from build123d import *

# Parameters (mm, degrees)
SKETCH2_R   = 9.525
SKETCH2_R_2 = 7.874


with BuildPart() as part:
    # Sweep1: sweep along a path in Sketch1
    with BuildLine(Plane.XY) as sweep1_path:
        Line((-82.715438584, 8.125207387), (-58.051554514, 8.125207387))
        ThreePointArc((-58.051554514, 8.125207387), (-44.819563376, 6.967558166), (-31.989619593, 3.529785091))
        Line((-31.989619593, 3.529785091), (83.882345193, -38.644161077))
        ThreePointArc((83.882345193, -38.644161077), (96.712288976, -42.081934153), (109.944280114, -43.239583374))
        Line((109.944280114, -43.239583374), (304.690435721, -43.239583374))
        ThreePointArc((304.690435721, -43.239583374), (324.412446958, -40.643131337), (342.790435721, -33.030719142))
        Line((342.790435721, -33.030719142), (363.602993383, -21.014583374))
    # Sketch2 → Sweep1 (sweep)
    with BuildSketch(Plane(origin=(-82.715438584, 8.125207387, 0), x_dir=(0, 0, -1), z_dir=(1, 0, 0))):
        Circle(SKETCH2_R)
        Circle(SKETCH2_R_2, mode=Mode.SUBTRACT)
    sweep(path=sweep1_path.line)


solid = part.part
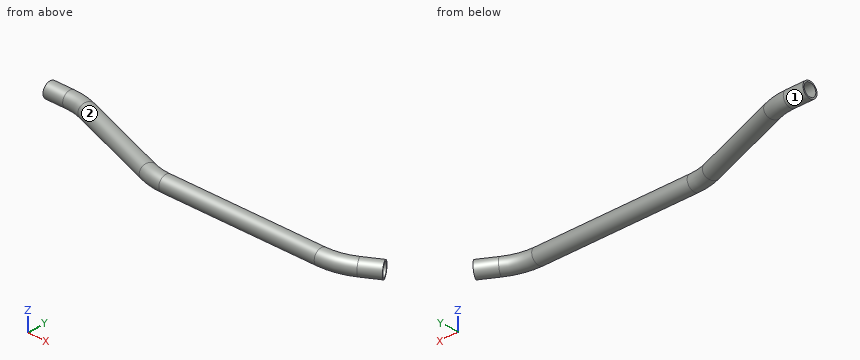
Read the model definition and answer for the solid it produces. Units are mm, in the model's axes. Face numbers are marked on the shaded views. Give positions to 0.01 mm unless a question says otherwise; leave off trailing zeros. Loops run counter-clockwise (first coordinate to the right, second up) from the corner with the lowest first, then second, coordinate; pieces in that order, holes last. Notation, with made-up numbers: (-31, -28.75) -> (-26, -28.75) arc R33 cw to (-26, 4.25) -> close; hole circle Ø7 at (0.5, 69). An arc over 180 degrees is marked (long way). Use a Markdown table: item, result.
Q1. Each of these flat-tipped pins is pushed along its axis until it touches: pin 1 (1.5 mm diameter, centred on x = 320.5, z = 0, fed in from -Y); pin 2 (2 mm diameter, centred on y = -41, z = -4, fed in from +X); pin 3 (1 mm diameter, centred on x = -22.5, z = 4.5, fed in from -Y). Where does it stop, or does it pass through?
Solved:
| item | result |
|---|---|
| pin 1 | stops at y = -51.43 |
| pin 2 | stops at x = 348.21 |
| pin 3 | stops at y = -9.18 |
Q2. Find the intervals of material crossed by line 1 along Y through (x, z) = (-72.25, 0); line 2 along Z through (x, y) = (111.5, -43); line 3 along Y through (x, z) = (262.5, 0), in increasing order.
Solved:
| item | result |
|---|---|
| line 1 | y = -1.4 to 0.25, 16 to 17.65 |
| line 2 | z = -9.52 to -7.87, 7.87 to 9.52 |
| line 3 | y = -52.76 to -51.11, -35.37 to -33.71 |
Q3. Section B-B, the plane x = 153.5 is taken. Determine the outline of the cut face in (y, z) (3 decimals).
Solved:
| item | result |
|---|---|
| outline | circle Ø19.05 at (-43.24, 0); hole circle Ø15.748 at (-43.24, 0) |
Q4. Determine the mould class of the marked faces 1 and 2 for opening direction X: pulls with the +X half, pulls with the -X half, needs draft (parallel to the pull), parting line crosses it, or undercut.
Solved:
| item | result |
|---|---|
| face 1 | needs draft |
| face 2 | undercut |
